Could you check a few things on this model? Use its own coordinates, in mm. Face numbers are marked on the shaded views. A direction names the side the tool comes from. Round coordinates to 2 decimals unless told otherwise and drop trailing zeros. Write each loop counter-clockwise with the first axis right and the second up, starting at its lowest first coordinate (ties: lowest second). Pieces come first, ordered by that corner, then holes.
```python
from build123d import *

# Parameters (mm, degrees)
POCKET_DEPTH = 1
CHAMFER_SIZE = 3.9


with BuildPart() as part:
    # Sketch004 (on XZ_Plane001 of Origin002) → Revolution001 (revolve)
    with BuildSketch(Plane.XZ):
        Polygon((6.5, 77), (12, 77), (12, 75), (8, 75), (8, 50), (12, 50), (12, 47), (6.5, 47), align=None)
    revolve(axis=Axis((0, 0, 0), (0, 0, 1)))

    # Sketch005 (on Face7 of Revolution001) → Pocket (cut)
    with BuildSketch(Plane(origin=(0, 0, 47), x_dir=(1, 0, 0), z_dir=(0, 0, -1))):
        with BuildLine():
            ThreePointArc((7.014806, 4.05), (0, 8.1), (-7.014806, 4.05))
            Line((-7.014806, 4.05), (-12, 4.05))
            Line((-12, 4.05), (-12, -4.05))
            Line((-12, -4.05), (-7.014806, -4.05))
            ThreePointArc((-7.014806, -4.05), (0, -8.1), (7.014806, -4.05))
            Line((7.014806, -4.05), (12, -4.05))
            Line((12, -4.05), (12, 4.05))
            Line((12, 4.05), (7.014806, 4.05))
        make_face()
    extrude(amount=-POCKET_DEPTH, mode=Mode.SUBTRACT)

    # Chamfer
    chamfer_edges = [part.edges().sort_by_distance(p)[0] for p in [
        (-8, 0, 75),
        (-8, 0, 50),
    ]]
    chamfer(chamfer_edges, length=CHAMFER_SIZE)


solid = part.part
```
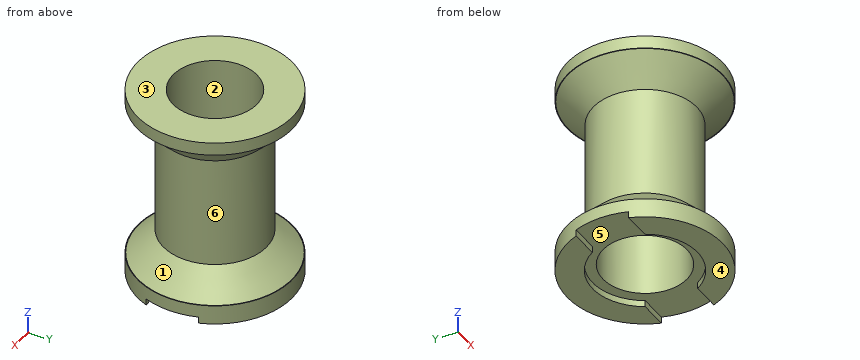
Q1. We'd pull the mould along Y, two halves only. Please class the marked faces 1, 2 and 3: pulls with the +Y half, pulls with the -Y half, needs draft (parallel to the pull), parting line crosses it, or undercut.
Q2. I'm going to push flat-ended pins straight in: pin 1 Ø1.5 at (x, z) = (6.5, 64) entering from +Y; pin 2 Ø0.5 at (x, z) = (9.5, 47.5) entering from -Y; pin 3 Ø8 at (x, z) = (-1.5, 60) entering from +Y. Where does each tip first touch, or does it pass through?
Q3. Imagine slicing it at B-B, the plane y = 0. Write out the boundary of the cut face in (x, z), then the cut area to 3 significant figures.
Q4. On a 3-axis mill with a long thin cutter (end or side, diameter ignored), from which of +Z, -Z, +X, -X, +Y, -Y can I reach the whole of each face in a straight line? I mean the marked faces 4, 5 and 6. Say none if no direction works.
Q5. Imagine slicing it at A-A, the plane x = 0. Write out the boundary of the cut face in (y, z), then the cut area to 3 significant figures.
Q6. Imagine slicing it at C-C, the plane z = 60.75. Write out the boundary of the cut face in (x, y), then the cut area to 3 significant figures.
Q7. If I drill on L1, parallel to Y at x = 0, z = 59.25; L2, parallel to Z at x = 3.75, y = -6.75; L3, parallel to Z at x = 8.5, y = 2.25, over which ranges is the centre line in solid material (lowest first)?
Results found:
1. face 1: parting line crosses it
1. face 2: undercut
1. face 3: needs draft
2. pin 1: stops at y = 5.56
2. pin 2: stops at y = -7.64
2. pin 3: stops at y = 8
3. outline: (-12, 48) - (-6.5, 48) - (-6.5, 77) - (-12, 77) - (-12, 75) - (-11.9, 75) - (-8, 71.1) - (-8, 53.9) - (-11.9, 50) - (-12, 50) - close; (6.5, 48) - (12, 48) - (12, 50) - (11.9, 50) - (8, 53.9) - (8, 71.1) - (11.9, 75) - (12, 75) - (12, 77) - (6.5, 77) - close
3. area: 149 mm2
4. face 4: -Z, +X, -X, +Y, -Y
4. face 5: -Z
4. face 6: none
5. outline: (-12, 47) - (-8.1, 47) - (-8.1, 48) - (-6.5, 48) - (-6.5, 77) - (-12, 77) - (-12, 75) - (-11.9, 75) - (-8, 71.1) - (-8, 53.9) - (-11.9, 50) - (-12, 50) - close; (6.5, 48) - (8.1, 48) - (8.1, 47) - (12, 47) - (12, 50) - (11.9, 50) - (8, 53.9) - (8, 71.1) - (11.9, 75) - (12, 75) - (12, 77) - (6.5, 77) - close
5. area: 157 mm2
6. outline: circle Ø16 at (0, 0); hole circle Ø13 at (0, 0)
6. area: 68.3 mm2
7. L1: y = -8 to -6.5, 6.5 to 8
7. L2: z = 48 to 77
7. L3: z = 48 to 53.11, 71.89 to 77
